Check sheet for the modelled part. Datum: model origin and axes. Units: mm. A direction names the side the tool comes from. Give positions to 0.01 mm unless a question says otherwise; leave off trailing zeros. Write each loop counter-clockwise with the first axis right and the second up, starting at its lowest first coordinate (ties: lowest second). Pieces come first, ordered by that corner, then holes. Notation, with made-up numbers: (87.25, -30) -> (92.25, -30) arc R22 ccw to (92.25, -17) -> close; hole circle Ø4 at (-37, -6). An arc over 180 degrees is marked (long way). Answer as a JSON object with one key per item and string values.
from build123d import *

# Parameters (mm, degrees)
BOSS_EXTRUDE1_DEPTH = 5
SKETCH2_R           = 1.5
CUT_EXTRUDE1_DEPTH  = 10


with BuildPart() as part:
    # Sketch1 → Boss-Extrude1 (new, symmetric)
    with BuildSketch(Plane.XY):
        with BuildLine():
            Line((-11.857417562, 2), (-11.857417562, 3.2))
            Line((-11.857417562, 3.2), (-1.857417562, 3.2))
            ThreePointArc((-1.857417562, 3.2), (3.7, 0), (-1.857417562, -3.2))
            Line((-1.857417562, -3.2), (-11.857417562, -3.2))
            Line((-11.857417562, -3.2), (-11.857417562, -2))
            Line((-11.857417562, -2), (-2.291287847, -2))
            Line((-2.291287847, -2), (-2.291287847, -1))
            ThreePointArc((-2.291287847, -1), (2.5, 0), (-2.291287847, 1))
            Line((-2.291287847, 1), (-2.291287847, 2))
            Line((-2.291287847, 2), (-11.857417562, 2))
        make_face()
    extrude(amount=BOSS_EXTRUDE1_DEPTH, both=True)

    # Sketch2 → Cut-Extrude1 (cut)
    with BuildSketch(Plane(origin=(0, 3.2, 0), x_dir=(1, 0, 0), z_dir=(0, 1, 0))):
        with Locations(Location((-6.857417562, 0, 0), (0, 0, 180))):
            Circle(SKETCH2_R)
        with BuildLine():
            Line((-6.857417562, 5), (-12.857417562, 5))
            Line((-12.857417562, 5), (-12.857417562, -5))
            Line((-12.857417562, -5), (-6.857417562, -5))
            ThreePointArc((-6.857417562, -5), (-11.857417562, 0), (-6.857417562, 5))
        make_face()
    extrude(amount=-CUT_EXTRUDE1_DEPTH, mode=Mode.SUBTRACT)


solid = part.part
1. Sectioned sample at C-C, the plane x = -7.5. Enter the section's corners in (y, z), plus the area to 3 significant figures.
Determined:
{"outline": "(-3.2, -4.96) -> (-2, -4.96) -> (-2, -1.36) -> (-3.2, -1.36) -> close; (-3.2, 1.36) -> (-2, 1.36) -> (-2, 4.96) -> (-3.2, 4.96) -> close; (2, -4.96) -> (3.2, -4.96) -> (3.2, -1.36) -> (2, -1.36) -> close; (2, 1.36) -> (3.2, 1.36) -> (3.2, 4.96) -> (2, 4.96) -> close", "area": "17.3 mm^2"}
2. Sectioned sample at D-D, the plane z = -3.75. Enter the section's corners in (x, y).
Determined:
{"outline": "(-10.16, -3.2) -> (-1.86, -3.2) arc R3.7 ccw (long way) to (-1.86, 3.2) -> (-10.16, 3.2) -> (-10.16, 2) -> (-2.29, 2) -> (-2.29, 1) arc R2.5 cw (long way) to (-2.29, -1) -> (-2.29, -2) -> (-10.16, -2) -> close"}
3. Mould release check, pull along X, two halves, no side actions. Record for faces 4 (the face through (2.5, -0.1, 0.1)), 5 (the face through (-11.856, 2.608, 0.11)), 6 (the face through (-5, 3.2, 0)): released by +X, released by -X, zero draft, split by the parting line, or undercut.
Determined:
{"face 4": "undercut", "face 5": "released by -X", "face 6": "zero draft"}
4. Sectioned sample at A-A, the plane x = 0. Enter the section's corners in (y, z), plus the area to 3 significant figures.
Determined:
{"outline": "(-3.7, -5) -> (-2.5, -5) -> (-2.5, 5) -> (-3.7, 5) -> close; (2.5, -5) -> (3.7, -5) -> (3.7, 5) -> (2.5, 5) -> close", "area": "24.0 mm^2"}
5. Sectioned sample at B-B, the plane z = 0. Enter the section's corners in (x, y).
Determined:
{"outline": "(-11.86, -3.2) -> (-8.36, -3.2) -> (-8.36, -2) -> (-11.86, -2) -> close; (-11.86, 2) -> (-8.36, 2) -> (-8.36, 3.2) -> (-11.86, 3.2) -> close; (-5.36, -3.2) -> (-1.86, -3.2) arc R3.7 ccw (long way) to (-1.86, 3.2) -> (-5.36, 3.2) -> (-5.36, 2) -> (-2.29, 2) -> (-2.29, 1) arc R2.5 cw (long way) to (-2.29, -1) -> (-2.29, -2) -> (-5.36, -2) -> close"}
6. Go/stop test with flat-tipped pins: P1, Ø4, axis at x = -6.86, z = 0, coming from the +Y side; P2, Ø2, axis at x = -5, z = 1, coming from the -Y side; P3, Ø1.1, axis at y = 1.5, z = -0.5, coming from the -X side. Record where each tip stops, or that it passes through.
Determined:
{"P1": "y = 3.2", "P2": "y = -3.2", "P3": "x = -11.85"}
7. Access from +Z, -Z, +X, -X, +Y, -Y to the whole of each face (thin tool, end or side, straight path). Record for faces 1 (the face through (-2, -2, -5)), 2 (the face through (-5.7, -3.2, 1.2)), 3 (the face through (-5, 2, 0)).
Determined:
{"face 1": "-Z, +X, -X, +Y, -Y", "face 2": "+Z, -Z, -X, -Y", "face 3": "+Z, -Z, -X"}
8. Scan lines: L1, parallel to Y at x = -10.5, z = -3.25; L2, parallel to Y at x = -2, z = 4; L3, parallel to X at y = 0.25, z = 4.75. Record each from-to range of solid material in increasing order. Write a range as [from, to].
Determined:
{"L1": "[-3.2, -2], [2, 3.2]", "L2": "[-3.2, -1.5], [1.5, 3.2]", "L3": "[2.49, 3.69]"}
